Source: three-view drawing plus pictorial views. Frame: mm from the lowest corner of the part. A direction names the side the tool comes from. Give positions to 0.01 mm unless a question says otherwise; leave off trailing zeros. Loops run counter-clockwise (first coordinate to the right, second up) from the corner with the lowest first, then second, coordinate; pieces in that order, holes last. Notation, with made-up numbers: M 27,87 L 81,87 A8 cw 81,91 Z; hole C -13,64.5 d5. An arc over 180 degrees is marked long. Write item = value, one per line.
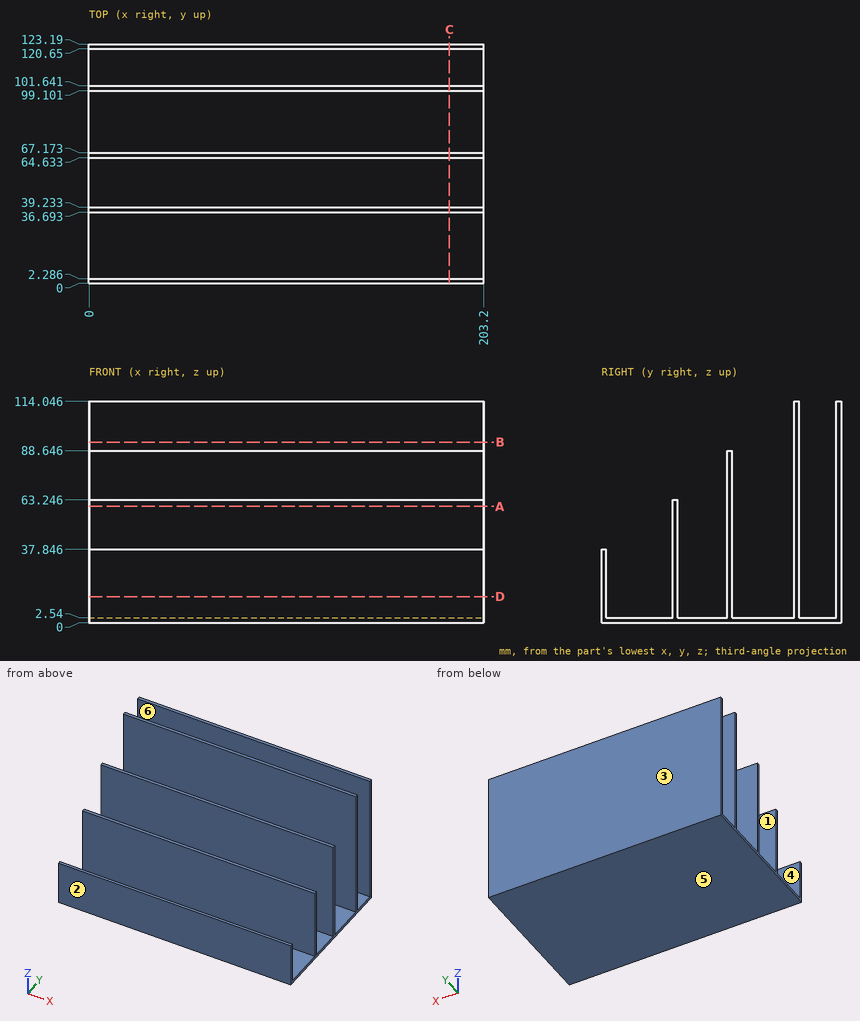
1. Cut plane B-B, the plane z = 93. Return the cut outline in (x, y), then the cut area to 3 significant figures.
Derived:
outline = M 0,99.1 L 203.2,99.1 L 203.2,101.64 L 0,101.64 Z; M 0,120.65 L 203.2,120.65 L 203.2,123.19 L 0,123.19 Z
area = 1,030 mm²
2. Cut plane C-C, the plane x = 185.5. Return the cut outline in (y, z), then the cut area to 3 significant figures.
Derived:
outline = M 0,0 L 123.19,0 L 123.19,114.05 L 120.65,114.05 L 120.65,2.54 L 101.64,2.54 L 101.64,114.05 L 99.1,114.05 L 99.1,2.54 L 67.17,2.54 L 67.17,88.65 L 64.63,88.65 L 64.63,2.54 L 39.23,2.54 L 39.23,63.25 L 36.69,63.25 L 36.69,2.54 L 2.29,2.54 L 2.29,37.85 L 0,37.85 Z
area = 1,330 mm²
3. Material intervals for probe 1 along Y at (x, z) = (76.5, 35.5); probe 2 along Y at (x, z) = (112.5, 39); probe 3 along Y at (x, z) = (174.5, 89.5), sorted ascending. Write a range as from..to.
Derived:
probe_1 = 0..2.29, 36.69..39.23, 64.63..67.17, 99.1..101.64, 120.65..123.19
probe_2 = 36.69..39.23, 64.63..67.17, 99.1..101.64, 120.65..123.19
probe_3 = 99.1..101.64, 120.65..123.19
4. Cut plane D-D, the plane z = 13.5. Return the cut outline in (x, y), then the cut area to 3 significant figures.
Derived:
outline = M 0,0 L 203.2,0 L 203.2,2.29 L 0,2.29 Z; M 0,36.69 L 203.2,36.69 L 203.2,39.23 L 0,39.23 Z; M 0,64.63 L 203.2,64.63 L 203.2,67.17 L 0,67.17 Z; M 0,99.1 L 203.2,99.1 L 203.2,101.64 L 0,101.64 Z; M 0,120.65 L 203.2,120.65 L 203.2,123.19 L 0,123.19 Z
area = 2,530 mm²
5. Cut plane A-A, the plane z = 60. Return the cut outline in (x, y).
Derived:
outline = M 0,36.69 L 203.2,36.69 L 203.2,39.23 L 0,39.23 Z; M 0,64.63 L 203.2,64.63 L 203.2,67.17 L 0,67.17 Z; M 0,99.1 L 203.2,99.1 L 203.2,101.64 L 0,101.64 Z; M 0,120.65 L 203.2,120.65 L 203.2,123.19 L 0,123.19 Z
6. Pull-direction query (Y, two-part tool) for the marked faces 1, 2, 3 and 4; classes: +Y half, -Y half, draft (parallel to the pull), parting line (faces both ways), or undercut.
Derived:
face_1 = undercut
face_2 = -Y half
face_3 = +Y half
face_4 = undercut
7. First-contact query: pin 1 Ø6 at (x, y) = (180, 23.5) entering from +Z; pin 2 Ø1 at (x, z) = (170.5, 68.5) entering from -Y; pin 3 Ø10 at (x, y) = (83.5, 62.5) entering from +Z. Flat tips, straight axial feed; report the tip coordinate or a pass-through.
Derived:
pin_1 = 2.54
pin_2 = 64.63
pin_3 = 88.65
8. Reachability of the marked faces 5 and 6 from +Z, -Z, +X, -X, +Y, -Y: full face, straight path, thin tool, end or side. Return the list, or none.
Derived:
face_5 = -Z, +X, -X, +Y, -Y
face_6 = +Z, +X, -X
